Could you check a few things on this model? Use its own coordinates, in mm. A direction names the side the tool comes from. Coordinates: 2 decimals unless noted, no trailing zeros. Loops run counter-clockwise (first coordinate to the right, second up) from the corner with the lowest first, then second, coordinate; pieces in that order, holes last. Notation, with made-up numbers: M -37,48 L -12,48 A32 ccw -12,85 Z; hole C -9,78.5 d9. An arc over 180 degrees is marked long. Return JSON: item names as keys, results as strings. Group by question number.
from build123d import *

# Parameters (mm, degrees)
F2_R     = 3.175
F3_DEPTH = 6.35


with BuildPart() as f1:
    # F0 (on Front) → F1 (revolve)
    with BuildSketch(Plane.XZ):
        Polygon((26.67, -21.780774), (5.715, 48.069226), (3.175, 48.069226), (3.175, 41.719226), (0, 41.719226), (0, -21.780774), align=None)
    revolve(axis=Axis((0, 0, 9.969226), (0, 0, 1)))

    # F2 (on face) → F3 (cut)
    with BuildSketch(Plane(origin=(0, 0, -21.780774), x_dir=(1, 0, 0), z_dir=(0, 0, -1))):
        Circle(F2_R)
    extrude(amount=-F3_DEPTH, mode=Mode.SUBTRACT)


solid = f1.part
(1) Will these pins go through, and if not, where does the flat tip stop? P1, Ø1.5, axis at x = -3.5, z = 33, coming from the -Y side; P2, Ø1.5, axis at y = 0.5, z = 5, coming from the +X side; P3, Ø3, axis at x = 2.5, z = 17, coming from the +Y side.
(2) Imagine slicing it at D-D, the plane z = 22. Write out the boundary of the cut face in (x, y), then the cut area to 3 significant figures.
(3) Imagine slicing it at C-C, the plane z = 13.5. Write out the boundary of the cut face in (x, y).
(4) For faces 1 (the face through (0, -6, -21.781)), 2 (the face through (-0.69, 3.1, -18.65)), which set-ups out of +Z, -Z, +X, -X, +Y, -Y let a thin tool reach every point of the face, with its end or its side?
(5) Imagine slicing it at A-A, the plane x = 0. Write out the boundary of the cut face in (y, z) (3 decimals).
(6) We'd pull the mould along X, two halves only. Please class faces 3 (the face through (-10.886, -8.347, 21.394)), 4 (the face through (-0.69, -3.1, 44.85)), 5 (the face through (2.5, -2.5, 48.069)), 6 (the face through (0, 0, 41.719)): +X half, -X half, draft (parallel to the pull), parting line (faces both ways), or undercut.
(7) If I drill on L1, parallel to X at y = 0, z = -18.75 (3 decimals); L2, parallel to X at y = 0, z = -17.5 (3 decimals); L3, parallel to Y at x = 0, z = -17.25 (3 decimals), over which ranges is the centre line in solid material (lowest first)? Write a range as [from, to].
Checks:
{
 "1": {"P1": "y = -9.96", "P2": "x = 18.85", "P3": "y = 15.33"},
 "2": {"outline": "C 0,0 d27.07", "area": "576 mm²"},
 "3": {"outline": "C 0,0 d32.17"},
 "4": {"face 1": "-Z, +X, -X, +Y, -Y", "face 2": "-Z"},
 "5": {"outline": "M -26.67,-21.781 L -3.175,-21.781 L -3.175,-15.431 L 3.175,-15.431 L 3.175,-21.781 L 26.67,-21.781 L 5.715,48.069 L 3.175,48.069 L 3.175,41.719 L -3.175,41.719 L -3.175,48.069 L -5.715,48.069 Z"},
 "6": {"face 3": "parting line", "face 4": "undercut", "face 5": "draft", "face 6": "undercut"},
 "7": {"L1": "[-25.761, -3.175], [3.175, 25.761]", "L2": "[-25.386, -3.175], [3.175, 25.386]", "L3": "[-25.311, -3.175], [3.175, 25.311]"}
}
